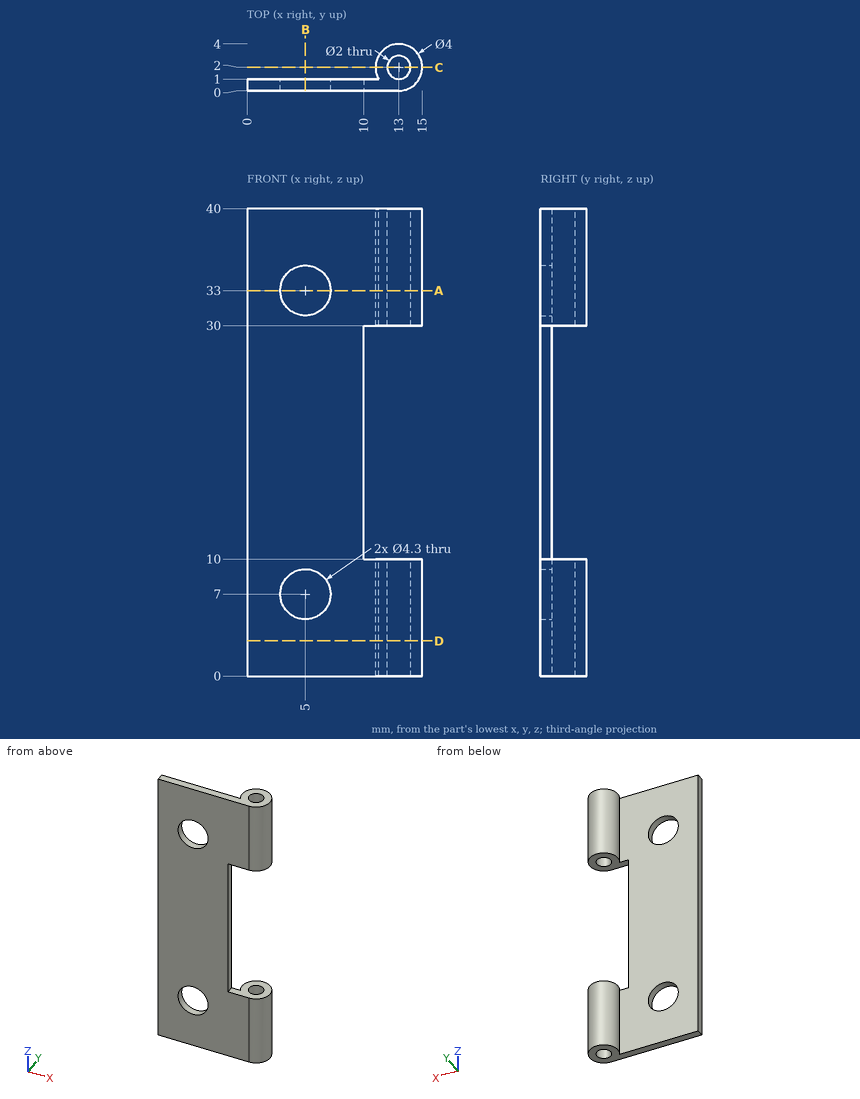
Drawing for the job (mm, zero at the part's lowest x, y, z). Coordinates: 2 decimals unless noted, no trailing zeros. Order: outer loops, then holes, each group sorted by start corner. A loop starts at its lowest first (then second) coordinate and runs counter-clockwise, first axis right, second up. Notation, with made-up numbers: (-33, 24.5) -> (-15, 24.5) arc R21 cw to (-15, 56.5) -> close; hole circle Ø9 at (-8.75, 17). An arc over 180 degrees is marked (long way). One line per item, written item: value.
(1) Slice it at D-D, the plane z = 3. List the corners of the cut face in (x, y).
Checked values:
outline: (0, 0) -> (13, 0) arc R2 ccw (long way) to (11.27, 1) -> (0, 1) -> close; hole circle Ø2 at (13, 2)
(2) Drop flat-ended pins along their axis: pin 1 Ø2 at (x, y) = (12.5, 2.5) entering from +Z; pin 2 Ø4 at (x, z) = (6, 28) entering from +Y; pin 3 Ø0.5 at (y, z) = (0.5, 17.5) entering from +X. Give the stop position or say it passes through.
Checked values:
pin 1: z = 40
pin 2: y = 1
pin 3: x = 10
(3) Slice it at B-B, the plane x = 5. List the corners of the cut face in (y, z).
Checked values:
outline: (0, 0) -> (1, 0) -> (1, 4.85) -> (0, 4.85) -> close; (0, 9.15) -> (1, 9.15) -> (1, 30.85) -> (0, 30.85) -> close; (0, 35.15) -> (1, 35.15) -> (1, 40) -> (0, 40) -> close
(4) Slice it at A-A, the plane z = 33. List the corners of the cut face in (x, y).
Checked values:
outline: (0, 0) -> (2.85, 0) -> (2.85, 1) -> (0, 1) -> close; (7.15, 0) -> (13, 0) arc R2 ccw (long way) to (11.27, 1) -> (7.15, 1) -> close; hole circle Ø2 at (13, 2)
(5) Probe line 1 (Z direction, x = 5, y = 0.4); line 2 (X direction, y = 2, z = 2); line 3 (Z direction, x = 14.75, y = 2). List the from-to ranges inside material, lowest first. Write a range as [from, to].
Checked values:
line 1: [0, 4.85], [9.15, 30.85], [35.15, 40]
line 2: [11, 12], [14, 15]
line 3: [0, 10], [30, 40]
(6) Slice it at C-C, the plane y = 2. List the corners of the cut face in (x, z).
Checked values:
outline: (11, 0) -> (12, 0) -> (12, 10) -> (11, 10) -> close; (11, 30) -> (12, 30) -> (12, 40) -> (11, 40) -> close; (14, 0) -> (15, 0) -> (15, 10) -> (14, 10) -> close; (14, 30) -> (15, 30) -> (15, 40) -> (14, 40) -> close
